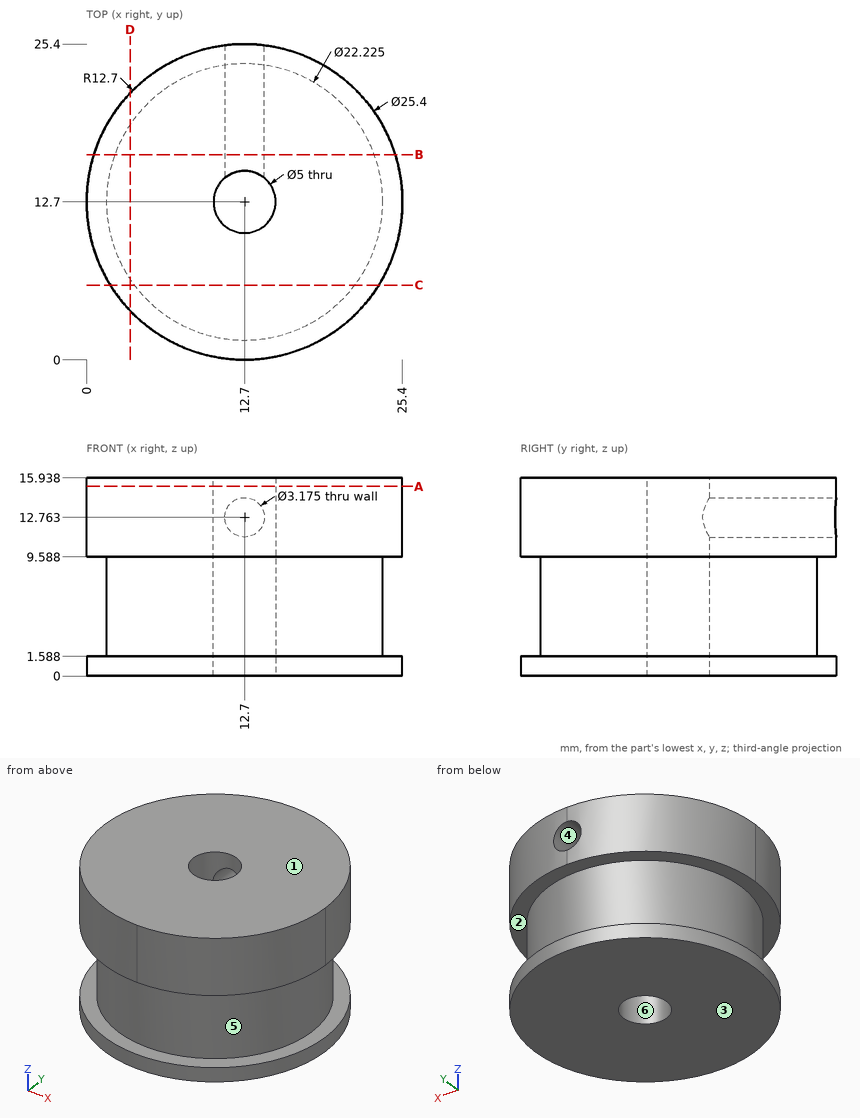
Could you check a few things on this drawing? It's one solid part, dimensions in mm from its lowest x, y, z. A direction names the side the tool comes from. Coordinates: 2 decimals unless noted, no trailing zeros. Order: outer loops, then holes, each group sorted by start corner. A loop starts at its lowest first (then second) coordinate and runs counter-clockwise, first axis right, second up.
1. I need wall thicknesses on line 1 (Y direction, x = 12.7, z = 9.5); line 2 (Z direction, x = 24.5, y = 14.5); line 3 (Y direction, x = 11.75, z = 4.75). Which ranges of each line are inside material? Lowest first, please.
2. For the marked faces 4, 5 and 6, which set-ups out of +Z, -Z, +X, -X, +Y, -Y let a thin tool reach every point of the face, with its end or its side?
3. If we section it at D-D (x = 3.5): Please give me the cut outline in (y, z) (1 decimal), then the cut area to 3 significant figures.
4. If we section it at C-C (y = 6): Please give me the cut outline in (x, z) (1 decimal).
5. If we section it at A-A (z = 15.25): Please give me the cut outline in (x, y), then the cut area to 3 significant figures.
6. Thinking about a two-plate mould opening in Z: for the marked faces 1, 2 and 3, which applies, +Z half, -Z half, draft (parallel to the pull), parting line (faces both ways), or undercut?
7. If we section it at B-B (y = 16.5): Please give me the cut outline in (x, z) (1 decimal).
8. I'm going to push flat-ended pins straight in: pin 1 (4 mm diameter, centred on x = 17.5, z = 6.5, fed in from +Y); pin 2 (4 mm diameter, centred on y = 12.5, z = 8, fed in from -X); pin 3 (1.9 mm diameter, centred on x = 12.7, z = 12.76, fed in from +Y); pin 4 (2 mm diameter, centred on x = 19.5, z = 3.5, fed in from +Y). Where does each tip first touch, or does it pass through?
Entries:
1. line 1: y = 1.59 to 10.2, 15.2 to 23.81
1. line 2: z = 0 to 1.59, 9.59 to 15.94
1. line 3: y = 1.63 to 10.39, 15.01 to 23.77
2. face 4: +Y
2. face 5: none
2. face 6: +Z, -Z
3. outline: (3.9, 0) - (21.5, 0) - (21.5, 1.6) - (18.9, 1.6) - (18.9, 9.6) - (21.5, 9.6) - (21.5, 15.9) - (3.9, 15.9) - (3.9, 9.6) - (6.5, 9.6) - (6.5, 1.6) - (3.9, 1.6) - close
3. area: 239 mm2
4. outline: (1.9, 0) - (23.5, 0) - (23.5, 1.6) - (21.6, 1.6) - (21.6, 9.6) - (23.5, 9.6) - (23.5, 15.9) - (1.9, 15.9) - (1.9, 9.6) - (3.8, 9.6) - (3.8, 1.6) - (1.9, 1.6) - close
5. outline: circle Ø25.4 at (12.7, 12.7); hole circle Ø5 at (12.7, 12.7)
5. area: 487 mm2
6. face 1: +Z half
6. face 2: undercut
6. face 3: -Z half
7. outline: (0.6, 0) - (24.8, 0) - (24.8, 1.6) - (23.1, 1.6) - (23.1, 9.6) - (24.8, 9.6) - (24.8, 15.9) - (0.6, 15.9) - (0.6, 9.6) - (2.3, 9.6) - (2.3, 1.6) - (0.6, 1.6) - close; hole circle Ø3.2 at (12.7, 12.8)
8. pin 1: stops at y = 23.45
8. pin 2: stops at x = 0
8. pin 3: stops at y = 10.39
8. pin 4: stops at y = 22.18
